The model under review builds one solid part; all positions refer to its coordinate system, in mm. Round coordinates to 2 decimals unless told otherwise and drop trailing zeros. Loops run counter-clockwise (first coordinate to the right, second up) from the corner with the lowest first, then second, coordinate; pieces in that order, holes last. Notation, with made-up numbers: (3.25, 59) -> (23.25, 59) arc R6 ccw to (23.25, 68) -> close; hole circle Ø8 at (11.25, -35). An arc over 180 degrees is marked (long way). Use a Markdown table: item, result. Add a question column.
1) Wall thickness on probe 1 along Y at (x, z) = (-21.5, 1858): over which ranges is the line inside the solid? List them lowest first.
2) Consider section B-B on z = 2120. Give the boundary of the cut face in (x, y).
3) Insertion check: pin 1 (12 mm diameter, centred on x = 30.5, y = -15, fed in from +Z). The pin has a flat end and moves straight along its axis. Give the tip position at first contact, or say it passes through.
4) Consider section C-C on x = 22. Give the boundary of the cut face in (y, z).
5) Consider section A-A on y = 11. Give the boundary of the cut face in (x, z), plus the area to 3 significant figures.
Autodesk Inventor part; units mm, degrees
ref_plane "Start Plane" through (0, 0, -80) normal (0, 0, 1) x (1, 0, 0)
ref_plane "End Plane" through (0, 0, 2418.3052) normal (0, 0, 1) x (1, 0, 0)
ref_plane "Work Plane4" through (1869.1883, -34, 509.1169) normal (0.7071, 0, 0.7071) x (0.7071, 0, -0.7071)
ref_plane "Start Plane" through (0, 0, -80) normal (0, 0, 1) x (1, 0, 0)
ref_plane "End Plane" through (0, 0, 2418.3052) normal (0, 0, 1) x (1, 0, 0)
sketch "Sketch" plane through (0, 0, 0) normal (0, 0, 1) x (1, 0, 0)
  line L0 (-40, -34) -> (-40, 34)
  line L1 (-34, 40) -> (34, 40)
  line L2 (40, 34) -> (40, -34)
  line L3 (34, -40) -> (-34, -40)
  arc A0 (-40, -34) -> (-34, -40) centre (-34, -34) ccw
  arc A1 (40, 34) -> (34, 40) centre (34, 34) ccw
  arc A2 (-34, 40) -> (-40, 34) centre (-34, 34) ccw
  arc A3 (34, -40) -> (40, -34) centre (34, -34) ccw
  arc A4 (-34, 37) -> (-37, 34) centre (-34, 34) ccw
  line L4 (-34, 37) -> (34, 37)
  arc A5 (37, 34) -> (34, 37) centre (34, 34) ccw
  line L5 (37, 34) -> (37, -34)
  arc A6 (34, -37) -> (37, -34) centre (34, -34) ccw
  line L6 (34, -37) -> (-34, -37)
  arc A7 (-37, -34) -> (-34, -37) centre (-34, -34) ccw
  line L7 (-37, -34) -> (-37, 34)
  line L8 (0, 57.7397) -> (0, -57.7397) construction
  line L9 (-57.7397, 0) -> (57.7397, 0) construction
  dimension "d7" = 6
  dimension "d9" = 80
  dimension "d11" = 80
  dimension "d12" = 3
  dimension "d15" = 40
  dimension "d16" = 40
extrude "Body" add sketch "Sketch" along normal up to surface (2498.3052 mm away) from surface at -80
sketch "Sketch3" plane through (0, 0, 0) normal (0, 0, 1) x (1, 0, 0)
  line L0 (0, 0) -> (10, 0)
ref_plane "Work Plane3" through (0, 0, 0) normal (0, -1, 0) x (1, 0, 0)
ref_plane "Work Plane4" through (1869.1883, -34, 509.1169) normal (0.7071, 0, 0.7071) x (0.7071, 0, -0.7071)
split "Split1" plane through (1869.1883, -34, 509.1169) removes the side toward (0.7071, 0, 0.7071)
ref_plane "Work Plane5" through (808.5281, 34, -848.5281) normal (-0.7071, 0, -0.7071) x (-0.7071, 0, 0.7071)
split "Split2" plane through (808.5281, 34, -848.5281) removes the side toward (-0.7071, 0, -0.7071)
sketch "Sketch4" plane through (0, 0, 0) normal (0, -1, 0) x (1, 0, 0)
  line L0 (-2, -80) -> (12, -80)
  line L1 (-2, 2418.3052) -> (12, 2418.3052)
  dimension "d18" = 2498.3052
equation "\"d7\" = G_IR"
equation "\"d9\" = G_W"
equation "\"d11\" = G_H"
equation "\"d12\" = G_T"
equation "\"d15\" = 0.5 * d9"
equation "\"d16\" = 0.5 * d11"
equation "\"d3\" = G_L"
equation "\"G_W\" = 80"
equation "\"G_H\" = 80"
equation "\"G_T\" = 3"
equation "\"G_IR\" = 6"
equation "\"G_L\" = d18"
equation "\"G_OFFSET_END\" = 0"
equation "\"d14\" = G_OFFSET_END + B_L"
equation "\"B_L\" = 2418.30519"
properties part number "ISO 10799-2 - 80x80x3 - 2498.31" material "Steel, Mild"
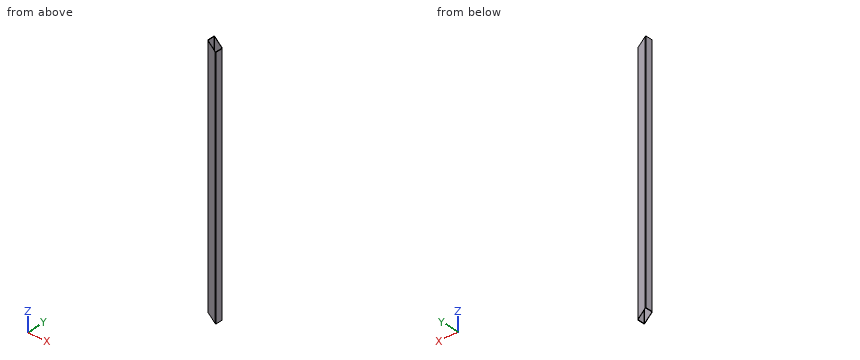
Result set:
| question | item | result |
|---|---|---|
| 1 | probe 1 | -40 to -37, 37 to 40 |
| 2 | outline | (-40, -34) arc R6 ccw to (-34, -40) -> (34, -40) arc R6 ccw to (40, -34) -> (40, 34) arc R6 ccw to (34, 40) -> (-34, 40) arc R6 ccw to (-40, 34) -> close; hole (-37, -34) arc R3 ccw to (-34, -37) -> (34, -37) arc R3 ccw to (37, -34) -> (37, 34) arc R3 ccw to (34, 37) -> (-34, 37) arc R3 ccw to (-37, 34) -> close |
| 3 | pin 1 | through |
| 4 | outline | (-40, -62) -> (-37, -62) -> (-37, 2356.31) -> (-40, 2356.31) -> close; (37, -62) -> (40, -62) -> (40, 2356.31) -> (37, 2356.31) -> close |
| 5 | outline | (-40, 0) -> (-37, -3) -> (-37, 2415.31) -> (-40, 2418.31) -> close; (37, -77) -> (40, -80) -> (40, 2338.31) -> (37, 2341.31) -> close |
| 5 | area | 14,500 mm2 |
